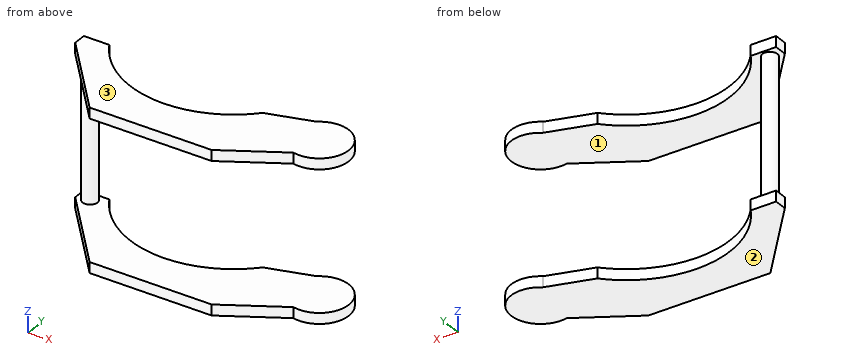
from build123d import *

# Parameters (mm, degrees)
BOSS_EXTRUDE1_DEPTH = 4
LPATTERN1_COUNT     = 2
LPATTERN1_PITCH     = 56
SKETCH2_R           = 2.789357995
BOSS_EXTRUDE2_DEPTH = 56


with BuildPart() as part:
    # Sketch1 → Boss-Extrude1 (new body)
    with BuildSketch(Plane.XY):
        with BuildLine():
            Line((-106.25, 0), (-96.75, 0))
            ThreePointArc((-96.75, 0), (-67.531499401, -19.450486235), (-34.603968254, -7.292366126))
            Line((-34.603968254, -7.292366126), (-17.738888889, -2.31334311))
            ThreePointArc((-17.738888889, -2.31334311), (-0.254682932, -8.640300495), (-13.492063492, -21.697850174))
            Line((-13.492063492, -21.697850174), (-35.416666667, -34.5))
            Line((-35.416666667, -34.5), (-80.952380952, -34.5))
            Line((-80.952380952, -34.5), (-106.25, -4.813953488))
            Line((-106.25, -4.813953488), (-106.25, 0))
        make_face()
    extrude(amount=BOSS_EXTRUDE1_DEPTH)


with BuildPart() as lpattern1_1:
    # LPattern1: pattern copy
    add(part.part.moved(Location(Vector(0, 0, 1) * (1 * LPATTERN1_PITCH))))


with BuildPart() as part_1:
    add(part.part)

    add(lpattern1_1.part)  # Boss-Extrude2 merges LPattern1_1
    # Sketch2 → Boss-Extrude2 (add)
    with BuildSketch(Plane.XY.offset(60)):
        with Locations((-101.5, -3.626457861)):
            Circle(SKETCH2_R)
    extrude(amount=-BOSS_EXTRUDE2_DEPTH)


solid = part_1.part
Model file for the job. Use its own axes, mm. Face numbers are marked on the shaded views. Coordinates: 2 decimals unless noted, no trailing zeros. Order: outer loops, then holes, each group sorted by start corner. A loop starts at its lowest first (then second) coordinate and runs counter-clockwise, first axis right, second up. Notation, with made-up numbers: M 3.5,11.25 L 43.5,11.25 A32 cw 43.5,48.25 Z; hole C -22.75,-1 d8. An arc over 180 degrees is marked long. Return JSON: item names as keys, results as strings.
1. Saw through at D-D (y = -18.5). Give the cut face in (x, z).
Ans:
{"outline": "M -94.59,0 L -72.64,0 L -72.64,4 L -94.59,4 Z; M -94.59,56 L -72.64,56 L -72.64,60 L -94.59,60 Z; M -53.4,0 L -2.96,0 L -2.96,4 L -53.4,4 Z; M -53.4,56 L -2.96,56 L -2.96,60 L -53.4,60 Z"}
2. Flat gauge pins, fed straight in: pin 1 (3 mm diameter, centred on y = -6.5, z = 32, fed in from +X); pin 2 (6 mm diameter, centred on x = -14.5, z = 9, fed in from -Y) (3 decimals). Where does each tip first touch, or does it go through?
Ans:
{"pin 1": "x = -99.07", "pin 2": "through"}
3. Saw through at A-A (x = -11). Give the cut face in (y, z).
Ans:
{"outline": "M -21.99,0 L 0,0 L 0,4 L -21.99,4 Z; M -21.99,56 L 0,56 L 0,60 L -21.99,60 Z"}
4. Saw through at B-B (y = -12). Give the cut face in (x, z).
Ans:
{"outline": "M -100.13,0 L -86.21,0 L -86.21,4 L -100.13,4 Z; M -100.13,56 L -86.21,56 L -86.21,60 L -100.13,60 Z; M -39.83,0 L -0.05,0 L -0.05,4 L -39.83,4 Z; M -39.83,56 L -0.05,56 L -0.05,60 L -39.83,60 Z"}
5. Pull direction Z, two halves, no side cores. Call the marked faces 1, 2 and 3: +Z half, -Z half, draft (parallel to the pull), parting line (faces both ways), or undercut.
Ans:
{"face 1": "undercut", "face 2": "-Z half", "face 3": "+Z half"}
6. Saw through at C-C (x = -64.5). Give the cut face in (y, z), and give its area (3 significant figures).
Ans:
{"outline": "M -34.5,0 L -19.69,0 L -19.69,4 L -34.5,4 Z; M -34.5,56 L -19.69,56 L -19.69,60 L -34.5,60 Z", "area": "119 mm^2"}
7. Drill centre lines: probe 1 along Z at (x, y) = (-28, -25); probe 2 along Y at (x, z) = (-18.5, 56.5). Where is each one in solid material? Low to high.
Ans:
{"probe 1": "0 to 4, 56 to 60", "probe 2": "-24.62 to -2.54"}
